Autodesk Inventor part; units mm, degrees
ref_plane "Start plane" through (0, 0, 50) normal (0, 0, 1) x (1, 0, 0)
ref_plane "End plane" through (0, 0, 1632) normal (0, 0, 1) x (1, 0, 0)
ref_plane "Work Plane4" through (9.2, 45, 1632) normal (0, 0, 1) x (1, 0, 0)
ref_plane "Start plane" through (0, 0, 50) normal (0, 0, 1) x (1, 0, 0)
ref_plane "End plane" through (0, 0, 1632) normal (0, 0, 1) x (1, 0, 0)
sketch "Sketch" plane through (0, 0, 0) normal (0, 0, 1) x (1, 0, 0)
  line L0 (-20, -13.4) -> (-20, 13.4)
  line L1 (-13.4, 20) -> (13.4, 20)
  line L2 (20, 13.4) -> (20, -13.4)
  line L3 (13.4, -20) -> (-13.4, -20)
  arc A0 (-20, -13.4) -> (-13.4, -20) centre (-13.4, -13.4) ccw
  arc A1 (-13.4, 20) -> (-20, 13.4) centre (-13.4, 13.4) ccw
  arc A2 (20, 13.4) -> (13.4, 20) centre (13.4, 13.4) ccw
  arc A3 (13.4, -20) -> (20, -13.4) centre (13.4, -13.4) ccw
  arc A4 (-13.4, 17) -> (-17, 13.4) centre (-13.4, 13.4) ccw
  line L4 (-13.4, 17) -> (13.4, 17)
  arc A5 (17, 13.4) -> (13.4, 17) centre (13.4, 13.4) ccw
  line L5 (17, 13.4) -> (17, -13.4)
  arc A6 (13.4, -17) -> (17, -13.4) centre (13.4, -13.4) ccw
  line L6 (13.4, -17) -> (-13.4, -17)
  arc A7 (-17, -13.4) -> (-13.4, -17) centre (-13.4, -13.4) ccw
  line L7 (-17, -13.4) -> (-17, 13.4)
  line L8 (0, 22.0873) -> (0, -22.0873) construction
  line L9 (-22.0873, 0) -> (22.0873, 0) construction
  dimension "d7" = 6.6
  dimension "d10" = 40
  dimension "d11" = 40
  dimension "d12" = 3
  dimension "d15" = 20
  dimension "d16" = 20
extrude "Body" add sketch "Sketch" along normal up to surface (1582 mm away) from surface at 50
sketch "Sketch3" plane through (0, 0, 0) normal (0, 0, 1) x (1, 0, 0)
  line L0 (0, 0) -> (10, 0)
ref_plane "Work Plane3" through (0, 0, 0) normal (0, -1, 0) x (1, 0, 0)
sketch "Sketch4" plane through (0, 0, 0) normal (0, -1, 0) x (1, 0, 0)
  line L0 (-2, 50) -> (12, 50)
  line L1 (-2, 1632) -> (12, 1632)
  dimension "d18" = 1582
ref_plane "Work Plane4" through (9.2, 45, 1632) normal (0, 0, 1) x (1, 0, 0)
split "Split1" plane through (9.2, 45, 1632) removes the side toward (0, 0, 1)
ref_plane "Work Plane5" through (-629.2, 45, 50) normal (0, 0, -1) x (-1, 0, 0)
split "Split2" plane through (-629.2, 45, 50) removes the side toward (0, 0, -1)
ref_plane "Work Plane6" through (-630.2, -705, 1632) normal (0, 0, 1) x (1, 0, 0)
split "Split3" plane through (-630.2, -705, 1632) removes the side toward (0, 0, 1)
equation "\"d7\" = G_IR"
equation "\"d10\" = G_H"
equation "\"d11\" = G_W"
equation "\"d12\" = G_T"
equation "\"d15\" = 0.5 * d10"
equation "\"d16\" = 0.5 * d11"
equation "\"d3\" = G_L"
equation "\"G_W\" = 40"
equation "\"G_H\" = 40"
equation "\"G_T\" = 3"
equation "\"G_IR\" = 6.6"
equation "\"G_L\" = d18"
equation "\"d14\" = G_OFFSET_END + B_L"
equation "\"B_L\" = 1682"
properties part number "DIN EN 10305-5 - 40 x 40 x 3  - 1582" material "Steel, Mild"
Read the model definition and answer for the solid it produces. Units are mm, in the model's axes. A direction names the side the tool comes from. Coordinates: 2 decimals unless noted, no trailing zeros. Write each loop counter-clockwise with the first axis right and the second up, starting at its lowest first coordinate (ties: lowest second). Pieces come first, ordered by that corner, then holes. Notation, with made-up numbers: (-9, -19.75) -> (45, -19.75) arc R22 cw to (45, -8.75) -> close; hole circle Ø1 at (-15, 54). An arc over 180 degrees is marked (long way). Answer as a JSON object with one key per item and string values.
Q1. Determine the mould class of faces 1 (the flat face through (-17, 0, 830)), 2 (the flat face through (-20, 0, 830)), 3 (the flat face through (20, 0, 830)) for opening direction X: pulls with the +X half, pulls with the -X half, needs draft (parallel to the pull), parting line crosses it, or undercut.
The answers:
{"face 1": "undercut", "face 2": "pulls with the -X half", "face 3": "pulls with the +X half"}
Q2. Consider line 1 (X direction, y = 5.5, z = 334.5); line 2 (X direction, y = 14, z = 1135.5). Determine where each line is inside the solid, lowest interval first. Write a range as [from, to].
The answers:
{"line 1": "x = [-20, -17], [17, 20]", "line 2": "x = [-19.97, -16.95], [16.95, 19.97]"}
Q3. A tool of negligible diameter and unlimited length cuts with its end or side. For faces 4 (the flat face through (0, -20, 830)), 5 (the flat face through (17, 0, 830)), from which of +Z, -Z, +X, -X, +Y, -Y can it reach the whole face along a straight path? Write none if from no direction.
The answers:
{"face 4": "+Z, -Z, +X, -X, -Y", "face 5": "+Z, -Z"}
Q4. The part is cut by section A-A on y = 3. Give the vertices of the cut face in (x, z).
The answers:
{"outline": "(-20, 50) -> (-17, 50) -> (-17, 1632) -> (-20, 1632) -> close; (17, 50) -> (20, 50) -> (20, 1632) -> (17, 1632) -> close"}
Q5. The part is cut by section C-C on z = 469. Give the vertices of the cut face in (x, y), then the cut area to 3 significant figures.
The answers:
{"outline": "(-20, -13.4) arc R6.6 ccw to (-13.4, -20) -> (13.4, -20) arc R6.6 ccw to (20, -13.4) -> (20, 13.4) arc R6.6 ccw to (13.4, 20) -> (-13.4, 20) arc R6.6 ccw to (-20, 13.4) -> close; hole (-17, -13.4) arc R3.6 ccw to (-13.4, -17) -> (13.4, -17) arc R3.6 ccw to (17, -13.4) -> (17, 13.4) arc R3.6 ccw to (13.4, 17) -> (-13.4, 17) arc R3.6 ccw to (-17, 13.4) -> close", "area": "418 mm2"}
